Autodesk Fusion 360 part; units mm, degrees
sketch "Sketch1" plane through (0, 0, 0) normal (0, 1, 0) x (1, 0, 0)
  line L0 (-9, 24) -> (9, 24)
  line L1 (9, 24) -> (9, -24)
  line L2 (9, -24) -> (-9, -24)
  line L3 (-9, -24) -> (-9, 24)
  line L4 (-9, 24) -> (9, -24) construction
  line L5 (9, 24) -> (-9, -24) construction
  dimension "d1" = 18
  dimension "d2" = 48
extrude "Extrude1" add sketch "Sketch1" against normal blind 2.5
sketch "Sketch2" plane through (0, 0, 0) normal (0, 1, 0) x (-1, 0, 0)
  line L0 (9, 24) -> (-9, 24)
  line L1 (-9, 24) -> (-9, -24)
  line L2 (-9, -24) -> (9, -24)
  line L3 (9, -24) -> (9, 24)
  line L4 (9, -19) -> (-9, -19)
  line L5 (-9, -19) -> (-9, 18)
  line L6 (-9, 18) -> (9, 18)
  line L7 (9, 18) -> (9, -19)
  dimension "d5" = 37
  dimension "d6" = 5
extrude "Extrude2" add sketch "Sketch2" along normal blind 3.5 contours L1 L3 L4 L5 L6 L7
sketch "Sketch3" plane through (0, 0, -24) normal (0, 0, -1) x (-1, 0, 0)
  line L0 (9, 0) -> (-9, 0)
  line L1 (-9, 0) -> (-9, -2.5)
  line L2 (-9, -2.5) -> (9, -2.5)
  line L3 (9, -2.5) -> (9, 0)
  circle A0 centre (0, 0) radius 5
  dimension "d9" = 10
extrude "Extrude3" add sketch "Sketch3" along normal blind 14 contours L0 L2 A0 | L0 A0 | L2 A0
fillet "Fillet1" radius 0.5 5 edges at (4.6616, -1.8081, -38) (0, 5, -24) (4.8296, -1.2941, -24) (0, -5, -24) (-4.8296, -1.2941, -24)
sketch "Sketch4" plane through (0, 0, 24) normal (0, 0, 1) x (1, 0, 0)
  line L0 (9, 0) -> (-9, 0)
  line L1 (-9, 0) -> (-9, -2.5)
  line L2 (-9, -2.5) -> (9, -2.5)
  line L3 (9, -2.5) -> (9, 0)
  circle A0 centre (0, 0) radius 1.5
  circle A1 centre (5.5, 0) radius 1.5
  circle A2 centre (-5.5, 0) radius 1.5
  point P0 (5.5, 0)
  point P1 (-5.5, 0)
  dimension "d13" = 3
extrude "Extrude4" add sketch "Sketch4" along normal blind 8 contours L0 A1 | L0 A1 | L0 A0 | L0 A0 | L0 A2 | L0 A2
extrude "Extrude5" add 3 faces at (5.8665, 0.3401, 24) (0.3665, 0.3401, 24) (-5.1335, 0.3401, 24) along direction (0, 0, -1) blind 1
sketch "Sketch5" plane through (0, 0, -24) normal (0, 0, -1) x (-1, 0, 0)
  arc A0 (-5.5, 0) -> (-4.899, -2.5) centre (0, 0) ccw
  line L0 (-5.5, 0) -> (-9, 0)
  line L1 (-9, 0) -> (-9, -2.5)
  line L2 (-9, -2.5) -> (-4.899, -2.5)
  circle A1 centre (-7, 0) radius 1.5
  circle A2 centre (7, 0) radius 1.5
  point P0 (-7, 0)
  point P1 (7, 0)
  dimension "d18" = 3
  dimension "d19" = 3
extrude "Extrude6" add sketch "Sketch5" along normal blind 7 contours L0 A1 | L0 A1 | A2
extrude "Extrude7" add 2 faces at (-7.3665, 0.4891, -24) (6.6335, 0.3401, -24) along direction (0, 0, 1) blind 2
Design review of the part built by this model. Coordinates are the model's own, in mm. A direction names the side the tool comes from. Give positions to 0.01 mm unless a question says otherwise; leave off trailing zeros. Loops run counter-clockwise (first coordinate to the right, second up) from the corner with the lowest first, then second, coordinate; pieces in that order, holes last. Notation, with made-up numbers: (61, 77) -> (117, 77) arc R25 cw to (117, 105) -> close; hole circle Ø8 at (57, 53.25). An arc over 180 degrees is marked (long way). One line per item, written item: value.
Q1. We need section A-A on x = 0. Give the boundary of the cut face in (y, z), and give its area (3 significant figures).
Numbers:
outline: (-5, -37.5) arc R0.5 ccw to (-4.5, -38) -> (4.5, -38) arc R0.5 ccw to (5, -37.5) -> (5, -24.5) arc R0.5 ccw to (4.5, -24) -> (0, -24) -> (0, -19) -> (3.5, -19) -> (3.5, 18) -> (0, 18) -> (0, 23) -> (1.5, 23) -> (1.5, 32) -> (-1.5, 32) -> (-1.5, 24) -> (-2.5, 24) -> (-2.5, -24) -> (-4.5, -24) arc R0.5 ccw to (-5, -24.5) -> close
area: 415 mm^2
Q2. For pin 1 Ø5 at (x, z) = (-2.5, 20) entering from +Y; pin 2 Ø2 at (x, y) = (6.5, -2.5) entering from -Z; pin 3 Ø0.9 at (x, y) = (-7.5, 0.5) entering from -Z, all flat-tipped, find the tip position at first contact; note any pin that passes through.
Numbers:
pin 1: stops at y = 3.5
pin 2: stops at z = -24
pin 3: stops at z = -31
Q3. Machinability: for faces 1 (the flat face through (-7, 1, -22)), 2 (the flat face through (7, 0, -31)), 3 (the cylindrical face through (7.325, 1.464, -26.437)), 4 (the cylindrical face through (6.19, 1.33, 27.44)), 5 (the flat face through (-7, 0, -31)), which of the approach directions +Z, -Z, +X, -X, +Y, -Y give a long, thin tool a straight path to every point of the face, cutting with its end or side? Answer none if there is none.
Numbers:
face 1: +X, -X, +Y
face 2: -Z, +X, +Y, -Y
face 3: -Z
face 4: +Z
face 5: -Z, -X, +Y, -Y
Q4. Draft analysis for pull direction X (two halves, no side actions). For faces 6 (the flat face through (0, -2.5, 0)), 7 (the cylindrical face through (-6.675, 1.464, -26.437)), 8 (the flat face through (9, 1, 0)), state which applies: pulls with the +X half, pulls with the -X half, needs draft (parallel to the pull), parting line crosses it, or undercut.
Numbers:
face 6: needs draft
face 7: undercut
face 8: pulls with the +X half
Q5. For L1, parallel to Z at x = -1, y = 1; L2, parallel to Z at x = 2.75, y = 2; L3, parallel to Z at x = -6.5, y = 1, list the stretches that pass through material, from the lowest coordinate up.
Numbers:
L1: z = -38 to -24, -19 to 18, 23 to 32
L2: z = -38 to -24, -19 to 18
L3: z = -31 to -22, -19 to 18, 23 to 32
Q6. We need section B-B on z = 0. Give the boundary of the cut face in (x, y).
Numbers:
outline: (-9, -2.5) -> (9, -2.5) -> (9, 3.5) -> (-9, 3.5) -> close
Q7. We need section C-C on z = 20. Give the boundary of the cut face in (x, y), and give its area (3 significant figures).
Numbers:
outline: (-9, -2.5) -> (9, -2.5) -> (9, 0) -> (-9, 0) -> close
area: 45.0 mm^2
